Source: CAD feature listing. Evaluate the final solid. Frame: model axes, mm. A direction names the side the tool comes from. Give positions to 0.01 mm unless a question says otherwise; leave off trailing zeros. Loops run counter-clockwise (first coordinate to the right, second up) from the corner with the lowest first, then second, coordinate; pieces in that order, holes last. Notation, with made-up numbers: (64, 27) - (93, 27) arc R27 ccw to (93, 53) - close; hole circle Ø1 at (-24.5, 26). An arc over 180 degrees is marked (long way). Put each result on its own line as item: value.
Solid Edge part; units mm, degrees
sketch "Sketch1" plane through (0, 0, 0) normal (0, 0, 1) x (1, 0, 0)
  line L0 (0, 0) -> (0, 2.75)
  line L1 (0, 2.75) -> (3, 2.75)
  line L2 (3, 2.75) -> (3, 1.75)
  line L3 (3, 1.75) -> (20.5, 1.75)
  line L4 (20.5, 1.75) -> (20.5, 1.5)
  line L5 (20.5, 1.5) -> (32.6935, 1.5)
  line L6 (32.6935, 1.5) -> (33, 1.1935)
  line L7 (33, 1.1935) -> (33, 0)
  line L8 (33, 0) -> (0, 0)
revolve "RevolvedProtrusion1" add sketch "Sketch1" angle 360 about axis through (33, 0, 0) along (-1, 0, 0)
cosmetic_thread "Thread1"
sketch "Sketch2" plane through (0, 0, 0) normal (1, 0, 0) x (0, 1, 0)
  line L0 (-0.7217, 1.25) -> (-1.4434, 0)
  line L1 (-1.4434, 0) -> (-0.7217, -1.25)
  line L2 (-0.7217, -1.25) -> (0.7217, -1.25)
  line L3 (0.7217, -1.25) -> (1.4434, 0)
  line L4 (1.4434, 0) -> (0.7217, 1.25)
  line L5 (0.7217, 1.25) -> (-0.7217, 1.25)
extrude "ExtrudedCutout_1" cut sketch "Sketch2" along normal blind 1.3
properties part number "CDQS12_CQ-M3x30L"
1) Pin query (flat end, axial travel): P1, Ø1, axis at x = 26, y = 0.5, coming from the +Z side; P2, Ø2, axis at x = 11, z = 0.5, coming from the -Y side. Return the tip coordinate at first contact, or that it passes through.
Check result:
P1: z = 1.5
P2: y = -1.75
2) Section query D-D, the plane x = 21. Output: boundary loops of the cut face in (y, z).
Check result:
outline: circle Ø3 at (0, 0)
3) Material intervals for line 1 along Y through (x, z) = (13, 0.9); line 2 along X through (y, z) = (1.1, -1.8); line 3 along X through (y, z) = (1.35, -1), sorted ascending. Write a range as [from, to].
Check result:
line 1: [-1.5, 1.5]
line 2: [0, 3]
line 3: [0, 20.5]
4) Section query B-B, the plane x = 14. Output: boundary loops of the cut face in (y, z).
Check result:
outline: circle Ø3.5 at (0, 0)
5) Mould query, pull axis Y, two halves, no side actions, for faces 1 (the cylindrical face through (26.68, -1.5, 0.07)), 2 (the flat face through (0.64, -1.08, 0.63)), 3 (the flat face through (3, 2, 0)), 4 (the flat face through (0.641, -1.088, -0.616)). Classes: pulls with the +Y half, pulls with the -Y half, needs draft (parallel to the pull), parting line crosses it, or undercut.
Check result:
face 1: parting line crosses it
face 2: undercut
face 3: needs draft
face 4: undercut
6) Section query A-A, the plane y = 0. Output: boundary loops of the cut face in (x, z).
Check result:
outline: (0, -2.75) - (3, -2.75) - (3, -1.75) - (20.5, -1.75) - (20.5, -1.5) - (32.69, -1.5) - (33, -1.19) - (33, 1.19) - (32.69, 1.5) - (20.5, 1.5) - (20.5, 1.75) - (3, 1.75) - (3, 2.75) - (0, 2.75) - (0, 1.25) - (1.3, 1.25) - (1.3, -1.25) - (0, -1.25) - close
7) Access query for faces 5 (the cylindrical face through (11.872, 1.617, -0.67)), 6 (the cylindrical face through (1.521, -0.596, -2.685)), 7 (the flat face through (0.64, 1.08, -0.63)). Directions: +Z, -Z, +X, -X, +Y, -Y. A direction counts if a zero-diameter tool reaches every point of the face in a straight line with its end or side. Return the directions, or none.
Check result:
face 5: +X
face 6: +X, -X
face 7: -X
8) Section query C-C, the plane z = 2.05. Output: boundary loops of the cut face in (x, y), plus the area to 3 significant figures.
Check result:
outline: (0, -1.83) - (3, -1.83) - (3, 1.83) - (0, 1.83) - close
area: 11.0 mm²
